Verification items for the finished model (mm, model axes). A direction names the side the tool comes from. Round coordinates to 2 decimals unless told otherwise and drop trailing zeros. Write each loop counter-clockwise with the first axis right and the second up, starting at its lowest first coordinate (ties: lowest second). Pieces come first, ordered by that corner, then holes. Notation, with made-up numbers: M 38,17.25 L 75,17.25 A28 cw 75,42.25 Z; hole C 65,4.5 d6. An arc over 180 degrees is marked long. Answer in a Markdown table with one row per item. Add a question column.
1. Set-up check for faces 4 (the flat face through (-10, 6.6, 2)), 5 (the flat face through (2.4, 0, 2.1)): record each of +Z, -Z, +X, -X, +Y, -Y from which the full face is reachable in a straight line by a thin tool's end or side.
2. Material ranges on probe 1 along X at (y, z) = (4, -5); probe 2 along X at (y, z) = (3, -6); probe 3 along Y at (x, z) = (-9.75, 4.25), recorded low to high.
3. Sectioned sample at D-D on z = -6. Record the cut outline in (x, y), plus the area to 3 significant figures.
4. Go/stop test with flat-tipped pins: pin 1 Ø1.5 at (x, y) = (7, 1) entering from +Z; pin 2 Ø2 at (x, y) = (-5.5, 7) entering from +Z; pin 3 Ø2 at (y, z) = (1.5, -6) entering from +X. Record where each tip stops, or that it passes through.
5. Sectioned sample at A-A on z = 0. Record the cut outline in (x, y), plus the area to 3 significant figures.
6. Draft check along X on faces 1 (the flat face through (-2.3, 8.6, 2.3)), 2 (the cylindrical face through (7.5, 4.24, -0.07)), 3 (the cylindrical face through (-9.76, 3.25, -2.17)). Enter one of: pulls with the +X half, pulls with the -X half, needs draft (parallel to the pull), parting line crosses it, or undercut.
7. Sectioned sample at C-C on x = 5. Record the cut outline in (y, z).
8. Sectioned sample at B-B on y = 5.25. Record the cut outline in (x, z), plus the area to 3 significant figures.
```python
from build123d import *

# Parameters (mm, degrees)
SKETCH_1_R               = 10
SKETCH_1_R_2             = 3
EXTRUDE_1_DEPTH          = 6.6
SKETCH_2_R               = 11
SKETCH_2_R_2             = 3
EXTRUDE_2_DEPTH          = 2
CUT_EXTRUDE_1_REACH      = 19.775
SKETCH_3_R               = 1.5
PATTERN_CIRCULAR_1_COUNT = 4


with BuildPart() as part:
    # 草图1 → 凸台-拉伸1 (new body)
    with BuildSketch(Plane(origin=(0, 0, 0), x_dir=(1, 0, 0), z_dir=(0, 1, 0))):
        with Locations(Location((0, 0, 0), (0, 0, 270))):
            Circle(SKETCH_1_R)
        with Locations(Location((0, 0, 0), (0, 0, 270))):
            Circle(SKETCH_1_R_2, mode=Mode.SUBTRACT)
    extrude(amount=EXTRUDE_1_DEPTH)

    # 草图2 → 凸台-拉伸2 (add)
    with BuildSketch(Plane(origin=(0, 6.6, 0), x_dir=(1, 0, 0), z_dir=(0, 1, 0))):
        with Locations(Location((0, 0, 0), (0, 0, 270))):
            Circle(SKETCH_2_R)
        with Locations(Location((0, 0, 0), (0, 0, 270))):
            Circle(SKETCH_2_R_2, mode=Mode.SUBTRACT)
    extrude(amount=EXTRUDE_2_DEPTH)

    # 草图3 → 切除-拉伸1 (cut, up to next)
    with BuildSketch(Plane.XZ, mode=Mode.PRIVATE) as cut_extrude_1_sk1:
        with Locations(Location((0, 6, 0), (0, 0, 270))):
            Circle(SKETCH_3_R)
    cut_extrude_1_tool1 = extrude(cut_extrude_1_sk1.sketch, amount=-CUT_EXTRUDE_1_REACH, mode=Mode.PRIVATE) & part.part
    cut_extrude_1 = cut_extrude_1_tool1.solids().sort_by_distance((0, 0, 6))[0]
    add(cut_extrude_1, mode=Mode.SUBTRACT)

    # 阵列(圆周)1: 切除-拉伸1 ×4 about axis
    pattern_circular_1_axis = Axis((0, 0, 0), (0, 1, 0))
    for i in range(1, PATTERN_CIRCULAR_1_COUNT):
        add(cut_extrude_1.rotate(pattern_circular_1_axis, i * 360 / PATTERN_CIRCULAR_1_COUNT), mode=Mode.SUBTRACT)


solid = part.part
```
Geometry check:
| question | item | result |
|---|---|---|
| 1 | face 4 | -Y |
| 1 | face 5 | +Z, -Z, +X, -X, -Y |
| 2 | probe 1 | x = -8.66 to -1.12, 1.12 to 8.66 |
| 2 | probe 2 | x = -8 to -1.5, 1.5 to 8 |
| 2 | probe 3 | y = 6.6 to 8.6 |
| 3 | outline | M -9.22,6.6 L -8,6.6 L -8,0 L -1.5,0 L -1.5,8.6 L -9.22,8.6 Z; M 1.5,0 L 8,0 L 8,6.6 L 9.22,6.6 L 9.22,8.6 L 1.5,8.6 Z |
| 3 | area | 117 mm2 |
| 4 | pin 1 | stops at z = 7.81 |
| 4 | pin 2 | stops at z = 10.04 |
| 4 | pin 3 | stops at x = 8.66 |
| 5 | outline | M -11,6.6 L -10,6.6 L -10,0 L -7.5,0 L -7.5,8.6 L -11,8.6 Z; M -4.5,0 L -3,0 L -3,8.6 L -4.5,8.6 Z; M 3,0 L 4.5,0 L 4.5,8.6 L 3,8.6 Z; M 7.5,0 L 10,0 L 10,6.6 L 11,6.6 L 11,8.6 L 7.5,8.6 Z |
| 5 | area | 72.8 mm2 |
| 6 | face 1 | needs draft |
| 6 | face 2 | undercut |
| 6 | face 3 | parting line crosses it |
| 7 | outline | M 0,-8.66 L 6.6,-8.66 L 6.6,-9.8 L 8.6,-9.8 L 8.6,-1.12 L 0,-1.12 Z; M 0,1.12 L 8.6,1.12 L 8.6,9.8 L 6.6,9.8 L 6.6,8.66 L 0,8.66 Z |
| 8 | outline | C 0,0 d20; hole C -6,0 d3; hole C 0,0 d6; hole C 0,-6 d3; hole C 0,6 d3; hole C 6,0 d3 |
| 8 | area | 258 mm2 |
